Geometry check sheet. Reference: the model listing, model coordinates, mm. A direction names the side the tool comes from. Round coordinates to 2 decimals unless told otherwise and drop trailing zeros. Write each loop counter-clockwise with the first axis right and the second up, starting at its lowest first coordinate (ties: lowest second). Pieces come first, ordered by that corner, then holes. Notation, with made-up numbers: M -10,30 L 2,30 A5 cw 2,39 Z; hole C 15.25,83 d1. An arc over 180 degrees is marked long. Put each result on its own line as item: value. Start each with the question number.
(1) Material ranges on probe 1 along X at (y, z) = (-3.9, 0); probe 2 along X at (y, z) = (-6.25, -7.5); probe 3 along X at (y, z) = (-3.35, 0), recorded low to high.
(2) Section check B-B on z = -8.5. Record the cut outline in (x, y).
(3) Tool access check on faces 4 (the flat face through (9.95, -5, 0)), 5 (the flat face through (5, -7, -2.8)), 6 (the flat face through (0, -6, 10)). Record the directions out of +Z, -Z, +X, -X, +Y, -Y that give a thin tool (end or side, any length) a straight path to the whole face; none if there is none.
(4) Section check D-D on y = -4.25. Record the cut outline in (x, z), then the cut area to 3 significant figures.
(5) Section check A-A on x = 5. Record the cut outline in (y, z).
(6) Gauge pin test, flat ends, axial feed: pin 1 (2.5 mm diameter, centred on x = 20, y = -7, fed in from -Z); pin 2 (3 mm diameter, centred on y = -6.5, z = 10.5, fed in from +X); pin 3 (0.9 mm diameter, centred on x = 20.5, y = -6.5, fed in from +Z). Record the tip position at first contact, or that the pin passes through.
(7) Mould release check, pull along Z, two halves, no side actions. Record for faces 1 (the flat face through (-3, -6, -12)), 2 (the flat face through (15.45, -5, 0)), 3 (the cylindrical face through (28.612, -5.653, 0.115)): pulls with the +Z half, pulls with the -Z half, needs draft (parallel to the pull), parting line crosses it, or undercut.
(8) Section check C-C on x = 16. Record the cut outline in (y, z), then the cut area to 3 significant figures.
Autodesk Inventor part; units mm, degrees
ref_plane "YZ Plane" through (0, 0, 0) normal (1, 0, 0) x (0, 1, 0)
ref_plane "XZ Plane" through (0, 0, 0) normal (0, 1, 0) x (-1, 0, 0)
ref_plane "XY Plane" through (0, 0, 0) normal (0, 0, 1) x (1, 0, 0)
ref_plane "Arbeitsebene1" through (-0.5, 0, -8) normal (0, -1, 0) x (1, 0, 0)
sketch "Skizze1" plane through (-0.5, 0, -8) normal (0, -1, 0) x (1, 0, 0)
  line L0 (-6.1, 20) -> (0.5, 20)
  line L1 (0.5, 20) -> (0.5, -4)
  line L2 (0.5, -4) -> (-6.1, -4)
  line L3 (-6.1, -4) -> (-6.1, 20)
  line L4 (0.5, 0) -> (32.9, 0)
  line L5 (0.5, 16) -> (34.9, 16)
  line L6 (0.5, 0) -> (34.9, 0)
  line L7 (34.9, 0) -> (34.9, 16)
  line L8 (34.9, 16) -> (0.5, 16)
  line L9 (0.5, 16) -> (0.5, 0)
  circle A0 centre (5.5, 8) radius 1.6
  circle A1 centre (5.5, 8) radius 1.6
  circle A2 centre (20.5, 8) radius 1.6
  circle A3 centre (20.5, 8) radius 1.6
  circle A4 centre (5.5, 8) radius 2.75
  circle A5 centre (20.5, 8) radius 2.75
  point P0 (0.5, 8)
  dimension "d0" = 5.5
  dimension "d1" = 5.5
extrude "Extrusion1" add sketch "Skizze1" along normal blind 10 contours L0 L1 L2 L3 | L5 L7 L6 L4 L1 | A4 | A5
ref_plane "Arbeitsebene2" through (-6.6, 0, -12) normal (-1, 0, 0) x (0, 0, 1)
sketch "Skizze2" plane through (-6.6, 0, -12) normal (-1, 0, 0) x (0, 0, 1)
  line L0 (0, -10) -> (4, -10)
  line L1 (0, -10) -> (24, -10)
  line L2 (24, -10) -> (24, -25)
  line L3 (24, -25) -> (0, -25)
  line L4 (0, -25) -> (0, -10)
  line L5 (0, 0) -> (0, -10)
  line L6 (0, 0) -> (4, 0)
  line L7 (0, -10) -> (2, -10)
  line L8 (2, -10) -> (2, 0)
  line L9 (2, 0) -> (0, 0)
  line L10 (0, 0) -> (0, -10)
  line L11 (4, 0) -> (4, -10)
  line L12 (4, -10) -> (20, -10)
  line L13 (20, -10) -> (20, -20)
  line L14 (20, -20) -> (4, -20)
  line L15 (4, -20) -> (4, -10)
  line L16 (4, -10) -> (5.5, -10)
  line L17 (5.5, -10) -> (5.5, -20)
  line L18 (5.5, -20) -> (4, -20)
  line L19 (4, -20) -> (4, -10)
  circle A0 centre (12, -25) radius 16.3478
  line L20 (12, -8.6522) -> (12, -5.6522)
  line L21 (12, -5.6522) -> (12, -3.6522)
  circle A1 centre (12, -25) radius 19.3478
  circle A2 centre (12, -25) radius 21.3478
  line L22 (4, -20) -> (20, -20)
  line L23 (20, -20) -> (20, 0)
  line L24 (20, 0) -> (4, 0)
  line L25 (4, 0) -> (4, -20)
  point P0 (12, 0)
  point P1 (18.5, -10)
  point P2 (20, -7.3836)
  point P3 (20, -5.2079)
  point P4 (4, -5.2079)
  point P5 (4, -7.3836)
  dimension "d4" = 15
  dimension "d5" = 16
  dimension "d6" = 10
  dimension "d7" = 1.5
  dimension "d14" = 3
  dimension "d15" = 2
extrude "Extrusion2" cut sketch "Skizze2" against normal up to surface (41 mm away) contours A0 L1
sketch "Skizze4" plane through (-0.5, -10, -8) normal (0, -1, 0) x (1, 0, 0)
  circle A0 centre (20.5, 8) radius 1.6
  circle A1 centre (20.5, 8) radius 2.8
  circle A2 centre (5.5, 8) radius 1.6
  circle A3 centre (5.5, 8) radius 2.8
  line L0 (7.1166, 10.8) -> (8.7332, 8)
  line L1 (8.7332, 8) -> (7.1166, 5.2)
  line L2 (7.1166, 5.2) -> (3.8834, 5.2)
  line L3 (3.8834, 5.2) -> (2.2668, 8)
  line L4 (2.2668, 8) -> (3.8834, 10.8)
  line L5 (3.8834, 10.8) -> (7.1166, 10.8)
  line L6 (22.1166, 10.8) -> (23.7332, 8)
  line L7 (23.7332, 8) -> (22.1166, 5.2)
  line L8 (22.1166, 5.2) -> (18.8834, 5.2)
  line L9 (18.8834, 5.2) -> (17.2668, 8)
  line L10 (17.2668, 8) -> (18.8834, 10.8)
  line L11 (18.8834, 10.8) -> (22.1166, 10.8)
  point P0 (0.5, 8)
  point P1 (5.5, 10.8)
  point P2 (20.5, 10.8)
  dimension "d29" = 5.6
  dimension "d30" = 5.6
extrude "Extrusion3" cut sketch "Skizze4" against normal blind 5 contours A0 | A1 | A1 L6 L7 | A1 L11 L6 | L7 L8 A1 | A1 L10 L11 | L8 L9 A1 | A1 L9 L10 | A2 | A3 | A3 L0 L1 | A3 L5 L0 | L1 L2 A3 | A3 L4 L5 | L2 L3 A3 | A3 L3 L4
extrude "Extrusion4" cut sketch "Skizze2" against normal blind 38 contours L11 A2 L21 A1 | A1 L21 A2 L23
extrude "Extrusion5" add sketch "Skizze2" against normal blind 32.5 contours L11 A2 L21 A1 | A1 L21 A2 L23
extrude "Extrusion6" cut sketch "Skizze2" against normal blind 22.05 contours L11 A2 L21 A1 | A1 L21 A2 L23
extrude "Extrusion7" add sketch "Skizze2" against normal blind 16.55 contours L11 A2 L21 A1 | A1 L21 A2 L23
extrude "Extrusion8" cut sketch "Skizze1" along normal blind 16.55 contours A0 | A2
extrude "Extrusion9" cut sketch "Skizze1" along normal blind 2 contours L0 L1 L2 L3 | L5 L7 L6 L4 L1 | A4 | A5
fillet "Rundung1" radius 0.5 9 edges at (-3.3, -10, 12) (0, -10, 10) (17.2, -10, 8) (34.4, -10, 7.25) (34.4, -8.6522, 0) (34.4, -10, -7.25) (17.2, -10, -8) (0, -10, -10) (-3.3, -10, -12)
properties part number "OBS-Displaymountadapter"
Answers follow:
1. probe 1: x = -6.6 to 3.4, 6.6 to 9.95, 15.45 to 18.4, 21.6 to 25.9, 31.4 to 34.4
1. probe 2: x = -6.6 to 9.95, 15.45 to 25.9, 31.4 to 34.4
1. probe 3: x = -6.6 to 3.4, 6.6 to 18.4, 21.6 to 34.4
2. outline: M -6.6,-10 L -0.5,-10 A0.5 ccw 0,-9.5 L 0,-2 L -6.6,-2 Z
3. face 4: none
3. face 5: -Y
3. face 6: +Z, +X, +Y, -Y
4. outline: M -6.6,-12 L 0,-12 L 0,-8 L 34.4,-8 L 34.4,8 L 0,8 L 0,12 L -6.6,12 Z; hole C 5,0 d3.2; hole M 9.95,-5.02 L 15.45,-5.02 L 15.45,5.02 L 9.95,5.02 Z; hole C 20,0 d3.2; hole M 25.9,-5.02 L 31.4,-5.02 L 31.4,5.02 L 25.9,5.02 Z
4. area: 582 mm^2
5. outline: M -10,-7.5 A0.5 ccw -9.5,-8 L -2,-8 L -2,-1.6 L -5.72,-1.6 A19.35 cw -5.86,-2.8 L -8.89,-2.8 A16.35 cw -10,-6.5 Z; M -10,6.5 A16.35 cw -8.89,2.8 L -5.86,2.8 A19.35 cw -5.72,1.6 L -2,1.6 L -2,8 L -9.5,8 A0.5 ccw -10,7.5 Z
6. pin 1: stops at z = -8
6. pin 2: stops at x = 0
6. pin 3: stops at z = 8
7. face 1: pulls with the -Z half
7. face 2: undercut
7. face 3: parting line crosses it
8. outline: M -10,-7.5 A0.5 ccw -9.5,-8 L -2,-8 L -2,8 L -9.5,8 A0.5 ccw -10,7.5 L -10,6.5 A16.35 cw -10,-6.5 Z
8. area: 116 mm^2
